from build123d import *

# Parameters (mm, degrees)
SKETCH2_W           = 30
SKETCH2_H           = 30
BOSS_EXTRUDE2_DEPTH = 150
SKETCH3_R           = 2.5
CUT_EXTRUDE1_DEPTH  = 30
SKETCH4_OUTSIDE_W   = 63.176
SKETCH4_OUTSIDE_H   = 63.176
SKETCH4_OUTSIDE_R   = 12.5
CUT_EXTRUDE2_DEPTH  = 150
SKETCH5_R           = 11.5
CUT_EXTRUDE3_DEPTH  = 110
SKETCH7_W           = 12.5
SKETCH7_H           = 25
CUT_EXTRUDE4_DEPTH  = 30


with BuildPart() as part:
    # Sketch2 → Boss-Extrude2 (new body)
    with BuildSketch(Plane.XY):
        with Locations((-15, 15)):
            Rectangle(SKETCH2_W, SKETCH2_H)
    extrude(amount=BOSS_EXTRUDE2_DEPTH)

    # Sketch3 → Cut-Extrude1 (cut)
    with BuildSketch(Plane(origin=(0, 0, 0), x_dir=(0, 0, -1), z_dir=(1, 0, 0))):
        with Locations(Location((-135, 15, 0), (0, 0, 90))):
            Circle(SKETCH3_R)
    extrude(amount=-CUT_EXTRUDE1_DEPTH, mode=Mode.SUBTRACT)

    # Sketch4 outside → Cut-Extrude2 (cut)
    with BuildSketch(Plane.XY.offset(150)):
        with Locations((-15, 15)):
            Rectangle(SKETCH4_OUTSIDE_W, SKETCH4_OUTSIDE_H)
        with Locations((-15, 14.551643442)):
            Circle(SKETCH4_OUTSIDE_R, mode=Mode.SUBTRACT)
    extrude(amount=-CUT_EXTRUDE2_DEPTH, mode=Mode.SUBTRACT)

    # Sketch5 → Cut-Extrude3 (cut)
    with BuildSketch(Plane(origin=(0, 0, 0), x_dir=(-1, 0, 0), z_dir=(0, 0, -1))):
        with Locations((15, 14.551643442)):
            Circle(SKETCH5_R)
    extrude(amount=-CUT_EXTRUDE3_DEPTH, mode=Mode.SUBTRACT)

    # Sketch7 → Cut-Extrude4 (cut)
    with BuildSketch(Plane.XY.offset(150)):
        with Locations((-8.75, 14.551643442)):
            Rectangle(SKETCH7_W, SKETCH7_H)
    extrude(amount=-CUT_EXTRUDE4_DEPTH, mode=Mode.SUBTRACT)


solid = part.part
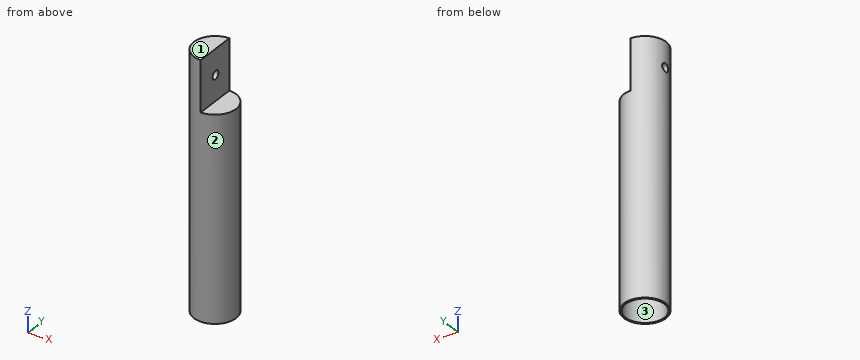
Design review of the part built by this model. Coordinates are the model's own, in mm. Face numbers are marked on the shaded views. Round coordinates to 2 decimals unless told otherwise and drop trailing zeros. Write each loop counter-clockwise with the first axis right and the second up, starting at its lowest first coordinate (ties: lowest second). Pieces come first, ordered by that corner, then holes. Notation, with made-up numbers: (56, -17.5) - (100, -17.5) arc R10 cw to (100, -3.5) - close; hole circle Ø11 at (48, 80). An arc over 180 degrees is marked (long way). Return JSON: item names as keys, results as strings. Group by question number.
Item 1: We need section C-C on x = -5. Write out the cut boundary in (y, z), and give its area (3 significant figures).
Item 2: We need section D-D on y = 6.25. Write out the cut boundary in (x, z).
Item 3: We need section B-B on z = 135. Write out the cut boundary in (x, y), and give its area (3 significant figures).
Item 4: Insertion check: P1, Ø5, axis at x = -19, z = 26.5, coming from the -Y side; P2, Ø1, axis at x = -13, y = 23.5, coming from the +Z side; P3, Ø12.5, axis at y = 12, z = 139.5, coming from the +X side. Each pin has a flat end and moves straight along its axis. Give the tip position at first contact, or say it passes through.
Item 5: We need section A-A on x = -23.75. Write out the cut boundary in (y, z).
Item 6: For probe 1 along X at (y, z) = (15.25, 35); probe 2 along Z at (x, y) = (-23, 15); probe 3 along Y at (x, z) = (-15, 83), list the stretches that pass through material, from the lowest coordinate up. Write a range as [from, to].
Item 7: The part is to be moulded in two halves that separate along Y. For the marked faces 1, 2 and 3, say which applies: pulls with the +Y half, pulls with the -Y half, needs draft (parallel to the pull), parting line crosses it, or undercut.
Model answer:
{
 "1": {"outline": "(7.05, 0) - (8.87, 0) - (8.87, 110) - (20.23, 110) - (20.23, 0) - (22.05, 0) - (22.05, 120) - (7.05, 120) - close", "area": "551 mm²"},
 "2": {"outline": "(-24.35, 0) - (-22.96, 0) - (-22.96, 110) - (-7.04, 110) - (-7.04, 0) - (-5.65, 0) - (-5.65, 120) - (-15, 120) - (-15, 150) - (-24.35, 150) - close"},
 "3": {"outline": "(-27.33, 12.5) arc R12.5 ccw to (-15, 2.05) - (-15, 12.5) - close; (-27.15, 17.5) - (-15, 17.5) - (-15, 27.05) arc R12.5 ccw to start", "area": "183 mm²"},
 "4": {"P1": "stops at y = 2.14", "P2": "stops at z = 120", "P3": "stops at x = -15"},
 "5": {"outline": "(5.62, 0) - (7.09, 0) - (7.09, 110) - (22.01, 110) - (22.01, 0) - (23.48, 0) - (23.48, 150) - (5.62, 150) - close; hole circle Ø5 at (15, 135)"},
 "6": {"probe 1": "x = [-27.48, -26.48], [-3.52, -2.52]", "probe 2": "z = [110, 132.5], [137.5, 150]", "probe 3": "y = [2.05, 3.05], [26.05, 27.05]"},
 "7": {"face 1": "needs draft", "face 2": "parting line crosses it", "face 3": "undercut"}
}
